Model file for the job. Use its own axes, mm. Face numbers are marked on the shaded views. A direction names the side the tool comes from. Round coordinates to 2 decimals unless told otherwise and drop trailing zeros. Order: outer loops, then holes, each group sorted by start corner. A loop starts at its lowest first (then second) coordinate and runs counter-clockwise, first axis right, second up. Notation, with made-up numbers: (36, -1.5) -> (83, -1.5) arc R13 ccw to (83, 14.5) -> close; hole circle Ø9 at (11.5, 70.25). An arc over 180 degrees is marked (long way). Answer as CSV lines item,"result".
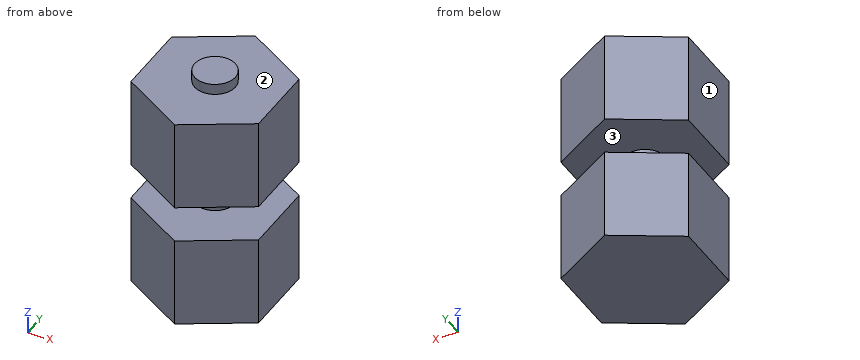
```python
from build123d import *

# Parameters (mm, degrees)
F0_R          = 1.4221963341
F1_DEPTH      = 6.35
F2_DEPTH      = 0.762
F2_DEPTH_BACK = 15.24
F3_START      = -8.89
F3_DEPTH      = 6.35


with BuildPart() as f1:
    # F0 (on Top) → F1 (new body)
    with BuildSketch(Plane.XY):
        Polygon((4.445, -2.5663219465), (4.445, 2.5663219465), (0, 5.1326438931), (-4.445, 2.5663219465), (-4.445, -2.5663219465), (0, -5.1326438931), align=None)
        Circle(F0_R, mode=Mode.SUBTRACT)
    extrude(amount=-F1_DEPTH)

    # F0 (on Top) → F2 (join, two sides)
    with BuildSketch(Plane.XY) as f2_sk:
        Circle(F0_R)
    extrude(amount=F2_DEPTH)
    extrude(f2_sk.sketch, amount=-F2_DEPTH_BACK)

    # F0 (on Top) → F3 (join)
    with BuildSketch(Plane.XY.offset(F3_START)):
        Polygon((4.445, -2.5663219465), (4.445, 2.5663219465), (0, 5.1326438931), (-4.445, 2.5663219465), (-4.445, -2.5663219465), (0, -5.1326438931), align=None)
        Circle(F0_R, mode=Mode.SUBTRACT)
    extrude(amount=-F3_DEPTH)


solid = f1.part
```
Q1. Tool access for the marked faces 1, 2 and 3: list every direction of +Z, -Z, +X, -X, +Y, -Y with a clear straight run to the whole face (end or side of a thin tool).
Checks:
face 1,"+Z, -Z, -X, +Y, -Y"
face 2,"+Z"
face 3,"none"
Q2. Saw through at B-B (x = 2). Write the cut outline in (y, z), plus the area to 3 significant figures.
Checks:
outline,"(-3.98, -15.24) -> (3.98, -15.24) -> (3.98, -8.89) -> (-3.98, -8.89) -> close; (-3.98, -6.35) -> (3.98, -6.35) -> (3.98, 0) -> (-3.98, 0) -> close"
area,"101 mm²"
Q3. Saw through at D-D (y = 0). Write the cut outline in (x, z) (3 decimals).
Checks:
outline,"(-4.445, -15.24) -> (4.445, -15.24) -> (4.445, -8.89) -> (1.422, -8.89) -> (1.422, -6.35) -> (4.445, -6.35) -> (4.445, 0) -> (1.422, 0) -> (1.422, 0.762) -> (-1.422, 0.762) -> (-1.422, 0) -> (-4.445, 0) -> (-4.445, -6.35) -> (-1.422, -6.35) -> (-1.422, -8.89) -> (-4.445, -8.89) -> close"
Q4. Flat gauge pins, fed straight in: pin 1 (1 mm diameter, centred on x = 2, z = -11.5, fed in from +Y); pin 2 (2 mm diameter, centred on x = -2, y = -1.5, fed in from +Z); pin 3 (6 mm diameter, centred on y = -3, z = -11.5, fed in from -X) (3 decimals). Where does each tip first touch, or does it go through?
Checks:
pin 1,"y = 4.27"
pin 2,"z = 0"
pin 3,"x = -4.445"
Q5. Saw through at A-A (y = -3). Write the cut outline in (x, z).
Checks:
outline,"(-3.69, -15.24) -> (3.69, -15.24) -> (3.69, -8.89) -> (-3.69, -8.89) -> close; (-3.69, -6.35) -> (3.69, -6.35) -> (3.69, 0) -> (-3.69, 0) -> close"
Q6. Saw through at C-C (z = -3.5). Write the cut outline in (x, y) (3 decimals).
Checks:
outline,"(-4.445, -2.566) -> (0, -5.133) -> (4.445, -2.566) -> (4.445, 2.566) -> (0, 5.133) -> (-4.445, 2.566) -> close"
Q7. Wall check: L1, parallel to Z at x = 0.25, y = 4.25; L2, parallel to Y at x = -1, z = -12; L3, parallel to X at y = 3.25, z = -2.25. Give the ranges that are in metal, low to high. Write a range as [from, to].
Checks:
L1,"[-15.24, -8.89], [-6.35, 0]"
L2,"[-4.56, 4.56]"
L3,"[-3.26, 3.26]"
